For this review, take the finished solid that the model builds, in its own axes (mm). Face numbers are marked on the shaded views. A direction names the side the tool comes from. Coordinates: 2 decimals unless noted, no trailing zeros. Loops run counter-clockwise (first coordinate to the right, second up) from the corner with the lowest first, then second, coordinate; pieces in that order, holes last. Notation, with made-up numbers: M -5.5,36.5 L 2.5,36.5 A21 cw 2.5,70.5 Z; hole C 87.5,61 d8. An arc over 180 degrees is marked long. Put each result on its own line as item: value.
```python
from build123d import *

# Parameters (mm, degrees)
SKETCH1_W               = 63.5
SKETCH1_H               = 20.066
BOSS_EXTRUDE1_DEPTH     = 6.35
SKETCH2_W               = 25.4
SKETCH2_H               = 20.066
BOSS_EXTRUDE2_DEPTH     = 3.175
SKETCH4_W               = 3.175
SKETCH4_H               = 20.066
BOSS_EXTRUDE3_DEPTH     = 19.05
SKETCH3_R               = 1.8
CUT_EXTRUDE1_DEPTH      = 61.325
CUT_EXTRUDE1_DEPTH_BACK = 4.175
SKETCH5_R               = 2.286
CUT_EXTRUDE2_DEPTH      = 7.35
SKETCH6_W               = 19.05
SKETCH6_H               = 20.066
CUT_EXTRUDE3_DEPTH      = 3.175
FILLET1_R               = 2.54
FILLET2_R               = 9.525


with BuildPart() as part:
    # Sketch1 → Boss-Extrude1 (new body)
    with BuildSketch(Plane.XY):
        Rectangle(SKETCH1_W, SKETCH1_H)
    extrude(amount=BOSS_EXTRUDE1_DEPTH)

    # Sketch2 → Boss-Extrude2 (add)
    with BuildSketch(Plane(origin=(31.75, 0, 0), x_dir=(0, 0, -1), z_dir=(1, 0, 0))):
        with Locations((-12.7, 0)):
            Rectangle(SKETCH2_W, SKETCH2_H)
    extrude(amount=-BOSS_EXTRUDE2_DEPTH)

    # Sketch4 → Boss-Extrude3 (add)
    with BuildSketch(Plane.XY.offset(6.35)):
        with Locations((7.9375, 0)):
            Rectangle(SKETCH4_W, SKETCH4_H)
    extrude(amount=BOSS_EXTRUDE3_DEPTH)

    # Sketch3 → Cut-Extrude1 (cut, two sides)
    with BuildSketch(Plane.ZY.offset(-28.575)) as cut_extrude1_sk:
        with Locations((15.875, 0)):
            Circle(SKETCH3_R)
    extrude(amount=CUT_EXTRUDE1_DEPTH, mode=Mode.SUBTRACT)
    extrude(cut_extrude1_sk.sketch, amount=-CUT_EXTRUDE1_DEPTH_BACK, mode=Mode.SUBTRACT)

    # Sketch5 → Cut-Extrude2 (cut, through all)
    with BuildSketch(Plane.XY.offset(6.35)):
        with Locations((-3.175, 0)):
            Circle(SKETCH5_R)
        with Locations((-25.4, 0)):
            Circle(SKETCH5_R)
    extrude(amount=-CUT_EXTRUDE2_DEPTH, mode=Mode.SUBTRACT)

    # Sketch6 → Cut-Extrude3 (cut)
    with BuildSketch(Plane.XY.offset(6.35)):
        with Locations((19.05, 0)):
            Rectangle(SKETCH6_W, SKETCH6_H)
    extrude(amount=-CUT_EXTRUDE3_DEPTH, mode=Mode.SUBTRACT)

    # Fillet1
    fillet1_edges = [part.edges().sort_by_distance(p)[0] for p in [
        (6.35, 0, 6.35),
        (28.575, 0, 3.175),
        (9.525, 0, 3.175),
    ]]
    fillet(fillet1_edges, radius=FILLET1_R)

    # Fillet2
    fillet2_edges = [part.edges().sort_by_distance(p)[0] for p in [
        (30.1625, 10.033, 25.4),
        (30.1625, -10.033, 25.4),
        (7.9375, -10.033, 25.4),
        (7.9375, 10.033, 25.4),
        (-31.75, -10.033, 3.175),
        (-31.75, 10.033, 3.175),
    ]]
    fillet(fillet2_edges, radius=FILLET2_R)


solid = part.part
```
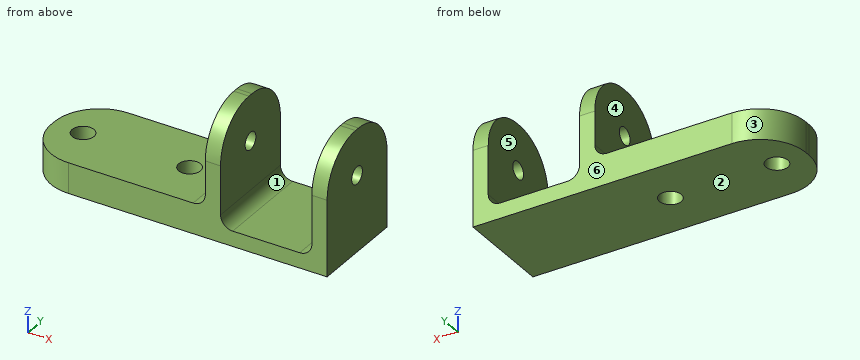
(1) For pin 1 (4 mm diameter, centred on x = -13, y = 4.5, fed in from +Z); pin 2 (4.5 mm diameter, centred on y = 0, z = 15.875, fed in from +X); pin 3 (1 mm diameter, centred on x = 23, z = 5.5, fed in from +Y); pin 4 (5 mm diameter, centred on y = 1, z = 14.5, fed in from -X), all flat-tipped, find the tip position at first contact; note any pin that passes through.
Determined:
pin 1: stops at z = 6.35
pin 2: stops at x = 31.75
pin 3: passes through
pin 4: stops at x = 6.35
(2) Add section B-B (x = -25.4). Write out the cut boundary in (y, z), plus the area to 3 significant figures.
Determined:
outline: M -9.49,0 L -2.29,0 L -2.29,6.35 L -9.49,6.35 Z; M 2.29,0 L 9.49,0 L 9.49,6.35 L 2.29,6.35 Z
area: 91.5 mm^2
(3) Wall thickness on line 1 along X through (y, z) = (7.25, 15) (3 decimals); line 2 along Z through (x, y) = (8.8, 0) (3 decimals); line 3 along Z through (x, y) = (-1, -2.5): over which ranges is each line inside the solid? List them lowest first. Write a range as [from, to].
Determined:
line 1: x = [6.35, 9.525], [28.575, 31.75]
line 2: z = [0, 14.075], [17.675, 25.4]
line 3: z = [0, 6.35]
(4) Draft analysis for pull direction X (two halves, no side actions). For the marked faces 1, 2 and 3, state which applies: +X half, -X half, draft (parallel to the pull), parting line (faces both ways), or undercut.
Determined:
face 1: undercut
face 2: draft
face 3: -X half
(5) Add section D-D (x = -8). Write out the cut boundary in (y, z), plus the area to 3 significant figures.
Determined:
outline: M -10.03,0 L 10.03,0 L 10.03,6.35 L -10.03,6.35 Z
area: 127 mm^2
(6) Add section A-A (z = 10.5). Write out the cut boundary in (x, y) (3 decimals).
Determined:
outline: M 6.35,-10.033 L 9.525,-10.033 L 9.525,10.033 L 6.35,10.033 Z; M 28.575,-10.033 L 31.75,-10.033 L 31.75,10.033 L 28.575,10.033 Z
(7) Add section C-C (y = -3.5). Write out the cut boundary in (x, z) (3 decimals), plus the area to 3 significant figures.
Determined:
outline: M -31.268,0 L 31.75,0 L 31.75,24.918 L 28.575,24.918 L 28.575,5.715 A2.54 cw 26.035,3.175 L 12.065,3.175 A2.54 cw 9.525,5.715 L 9.525,24.918 L 6.35,24.918 L 6.35,8.89 A2.54 cw 3.81,6.35 L -31.268,6.35 Z
area: 462 mm^2
(8) Tool access review of the marked faces 4, 5 and 6: name each direction out of +Z, -Z, +X, -X, +Y, -Y from which nothing blocks a thin tool from reaching the whole face with its end or side.
Determined:
face 4: +Z, -X, +Y, -Y
face 5: +Z, +Y, -Y
face 6: +Z, -Z, +X, -X, +Y
